Work out the finished part from the listing and answer in its coordinate system (mm). A direction names the side the tool comes from. Round coordinates to 2 decimals unless told otherwise and drop trailing zeros. Order: outer loops, then holes, each group sorted by start corner. A loop starts at its lowest first (then second) coordinate and runs counter-clockwise, first axis right, second up. Notation, with made-up numbers: M 71,-38 L 87,-38 A22 cw 87,-3 Z; hole C -32,10 d9. An arc over 180 degrees is marked long. Return JSON: item names as keys, results as strings.
from build123d import *

# Parameters (mm, degrees)
SKETCH_1_R          = 22.5
EXTRUDE_1_DEPTH     = 5
SKETCH_2_R          = 2
CUT_EXTRUDE_1_DEPTH = 33.210246817
SKETCH_3_R          = 55
EXTRUDE_2_DEPTH     = 5
SKETCH_4_R          = 5
CUT_EXTRUDE_2_DEPTH = 79.421935707
SKETCH_5_R          = 2
CUT_EXTRUDE_3_DEPTH = 78.942286341


with BuildPart() as part:
    # 草图1 → 凸台-拉伸1 (new body)
    with BuildSketch(Plane.XY):
        Circle(SKETCH_1_R)
    extrude(amount=EXTRUDE_1_DEPTH)

    # 草图2 → 切除-拉伸1 (cut, through all)
    with BuildSketch(Plane.XY.offset(5)):
        with Locations((17.25, 0)):
            Circle(SKETCH_2_R)
        with Locations((8.625, -14.938938215)):
            Circle(SKETCH_2_R)
        with Locations((-8.625, -14.938938215)):
            Circle(SKETCH_2_R)
        with Locations((-17.25, 0)):
            Circle(SKETCH_2_R)
        with Locations((-8.625, 14.938938215)):
            Circle(SKETCH_2_R)
        with Locations((8.625, 14.938938215)):
            Circle(SKETCH_2_R)
    extrude(amount=-CUT_EXTRUDE_1_DEPTH, mode=Mode.SUBTRACT)

    # 草图3 → 凸台-拉伸2 (add)
    with BuildSketch(Plane.XY.offset(5)):
        Circle(SKETCH_3_R)
    extrude(amount=EXTRUDE_2_DEPTH)

    # 草图4 → 切除-拉伸2 (cut, through all)
    with BuildSketch(Plane.XY.offset(10)):
        with Locations((45, 0)):
            Circle(SKETCH_4_R)
    extrude(amount=-CUT_EXTRUDE_2_DEPTH, mode=Mode.SUBTRACT)

    # 草图5 → 切除-拉伸3 (cut, through all)
    with BuildSketch(Plane(origin=(0, 0, 5), x_dir=(-1, 0, 0), z_dir=(0, 0, -1))):
        with Locations(Location((-8.625, 14.938938215, 0), (0, 0, 180))):
            Circle(SKETCH_5_R)
        with Locations(Location((-17.25, 0, 0), (0, 0, 180))):
            Circle(SKETCH_5_R)
        with Locations(Location((-8.625, -14.938938215, 0), (0, 0, 180))):
            Circle(SKETCH_5_R)
        with Locations(Location((8.625, -14.938938215, 0), (0, 0, 180))):
            Circle(SKETCH_5_R)
        with Locations(Location((17.25, 0, 0), (0, 0, 180))):
            Circle(SKETCH_5_R)
        with Locations(Location((8.625, 14.938938215, 0), (0, 0, 180))):
            Circle(SKETCH_5_R)
    extrude(amount=-CUT_EXTRUDE_3_DEPTH, mode=Mode.SUBTRACT)


solid = part.part
Item 1: Find section B-B (x = 17.5). Determine the outline of the cut face in (y, z).
Output:
{"outline": "M -52.14,5 L -14.14,5 L -14.14,0 L -1.98,0 L -1.98,10 L -52.14,10 Z; M 1.98,0 L 14.14,0 L 14.14,5 L 52.14,5 L 52.14,10 L 1.98,10 Z"}
Item 2: The mould has two halves that part along Y. Classify faces 3 (the cylindrical face through (-18.837, 1.217, 4.93)), 4 (the flat face through (0, 0, 0)), 5 (the cylindrical face through (40, 0, 8)), 6 (the cylindrical face through (10.382, -19.961, 2.465)): pulls with the +Y half, pulls with the -Y half, needs draft (parallel to the pull), parting line crosses it, or undercut.
Output:
{"face 3": "undercut", "face 4": "needs draft", "face 5": "undercut", "face 6": "parting line crosses it"}
Item 3: Find section C-C (z = 6.5). Determine the outline of the cut face in (x, y) (3 decimals), plus the area to 3 significant figures.
Output:
{"outline": "C 0,0 d110; hole C -17.25,0 d4; hole C -8.625,-14.939 d4; hole C -8.625,14.939 d4; hole C 8.625,-14.939 d4; hole C 8.625,14.939 d4; hole C 17.25,0 d4; hole C 45,0 d10", "area": "9,350 mm^2"}
Item 4: Consider line 1 along X through (y, z) = (-0.5, 7.5); line 2 along Z through (x, y) = (34.5, 4.5); line 3 along Y through (x, z) = (-19, 9.75). Determine where each line is inside the solid, lowest interval first. Write a range as [from, to].
Output:
{"line 1": "x = [-55, -19.19], [-15.31, 15.31], [19.19, 40.03], [49.97, 55]", "line 2": "z = [5, 10]", "line 3": "y = [-51.61, -0.97], [0.97, 51.61]"}
Item 5: Find section A-A (y = 0). Determine the outline of the cut face in (x, z).
Output:
{"outline": "M -55,5 L -22.5,5 L -22.5,0 L -19.25,0 L -19.25,10 L -55,10 Z; M -15.25,0 L 15.25,0 L 15.25,10 L -15.25,10 Z; M 19.25,0 L 22.5,0 L 22.5,5 L 40,5 L 40,10 L 19.25,10 Z; M 50,5 L 55,5 L 55,10 L 50,10 Z"}
Item 6: Find section D-D (x = 0). Determine the outline of the cut face in (y, z), plus the area to 3 significant figures.
Output:
{"outline": "M -55,5 L -22.5,5 L -22.5,0 L 22.5,0 L 22.5,5 L 55,5 L 55,10 L -55,10 Z", "area": "775 mm^2"}
Item 7: Each of these flat-tipped pins is pushed along its axis until it touches: pin 1 (11.5 mm diameter, centred on x = 45, y = 0, fed in from -Z); pin 2 (5 mm diameter, centred on x = -19, z = 6, fed in from -Y); pin 3 (1 mm diameter, centred on x = -24.5, z = 8.5, fed in from +Y). Where does it stop, or does it pass through?
Output:
{"pin 1": "stops at z = 5", "pin 2": "stops at y = -52.47", "pin 3": "stops at y = 49.49"}
Item 8: Which of the six approach directions +Z, -Z, +X, -X, +Y, -Y give full straight-line access (tool end or side, diameter ignored) to faces 1 (the flat face through (-1, -24, 5)), 2 (the cylindrical face through (-8.89, -16.92, 4.93))?
Output:
{"face 1": "-Z", "face 2": "+Z, -Z"}
